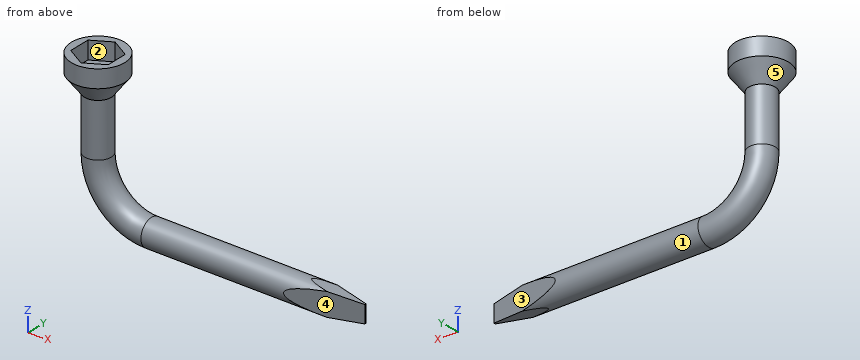
Autodesk Inventor part; units mm, degrees
ref_plane "YZ Plane" through (0, 0, 0) normal (1, 0, 0) x (0, 1, 0)
ref_plane "XZ Plane" through (0, 0, 0) normal (0, 1, 0) x (-1, 0, 0)
ref_plane "XY Plane" through (0, 0, 0) normal (0, 0, 1) x (1, 0, 0)
sketch "Эскиз1" plane through (0, 0, 0) normal (0, 1, 0) x (-1, 0, 0)
  line L0 (0, 0) -> (0, -30)
  line L1 (-30, -60) -> (-150, -60)
  arc A0 (-30, -60) -> (0, -30) centre (-30, -30) ccw
  point P0 (0, -60)
  dimension "d0" = 60
  dimension "d1" = 150
  dimension "d2" = 30
sketch "Эскиз2" plane through (0, 0, 0) normal (0, 0, 1) x (1, 0, 0)
  circle A0 centre (0, 0) radius 7.5
  dimension "d3" = 15
sweep "Сдвиг1" add profiles "Эскиз2" path "Эскиз1"
sketch "Эскиз3" plane through (0, 0, 0) normal (0, 1, 0) x (-1, 0, 0)
  line L0 (-120, -52.5) -> (-150, -55.1247)
  line L1 (-120, -67.5) -> (-150, -64.8753)
  line L2 (-150, -64.8753) -> (-150, -55.1247)
  line L3 (-150, -52.5) -> (-150, -67.5)
  line L4 (-120, -52.5) -> (-150.8821, -45.0422)
  line L5 (-150.8821, -45.0422) -> (-158.2895, -61.433)
  line L6 (-158.2895, -61.433) -> (-150, -78.5011)
  line L7 (-150, -78.5011) -> (-120, -67.5)
  point P0 (0, 0)
extrude "Выдавливание1" cut sketch "Эскиз3" against normal mid plane 40
sketch "Эскиз4" plane through (0, 0, 0) normal (0, 0, 1) x (1, 0, 0)
  line L0 (30, 7.5) -> (150, 7.5)
  line L1 (110, 7.5) -> (150.3931, 7.5) construction
  line L2 (30, -7.5) -> (150, -7.5)
  line L3 (110, 7.5) -> (159.1062, 20.8998)
  line L4 (159.1062, 20.8998) -> (172.0854, -18.5057)
  line L5 (172.0854, -18.5057) -> (124.0272, -32.5373)
  line L6 (124.0272, -32.5373) -> (110, -7.5)
  line L7 (110, 7.5) -> (150, 0.4469)
  line L8 (150, -5.6992) -> (150, 5.6992)
  line L9 (110, 7.5) -> (150.6171, 7.5) construction
  line L10 (110, -7.5) -> (150, -0.4469)
  line L11 (150, 0.4469) -> (150, -0.4469)
  point P0 (0, 0)
  dimension "d13" = 10
extrude "Выдавливание2" cut sketch "Эскиз4" against normal blind 120
sketch "Эскиз5" plane through (0, 0, 0) normal (0, 1, 0) x (-1, 0, 0)
  line L0 (0, 0) -> (0, 20)
  line L1 (0, 20) -> (15, 20)
  line L2 (15, 20) -> (15, 10)
  line L3 (7.5, 0) -> (-7.5, 0)
  line L4 (7.5, 0) -> (15, 10)
  dimension "d14" = 20
  dimension "d15" = 15
  dimension "d16" = 10
revolve "Вращение1" add sketch "Эскиз5" angle 360 about axis through (0, 0, 0) along (0, 0, 1)
sketch "Эскиз10" plane through (0, 0, 20) normal (0, 0, 1) x (1, 0, 0)
  line L0 (0, 12.1042) -> (10.4826, 6.0521)
  line L1 (10.4826, 6.0521) -> (10.4826, -6.0521)
  line L2 (10.4826, -6.0521) -> (0, -12.1042)
  line L3 (0, -12.1042) -> (-10.4826, -6.0521)
  line L4 (-10.4826, -6.0521) -> (-10.4826, 6.0521)
  line L5 (-10.4826, 6.0521) -> (0, 12.1042)
  point P0 (0, 0)
  point P1 (0, 0)
extrude "Выдавливание3" cut sketch "Эскиз10" against normal blind 10
properties part number "ключ" material "Сталь, гальванизированная"
Verification items for the finished model (mm, model axes). Face numbers are marked on the shaded views. A direction names the side the tool comes from. Round coordinates to 2 decimals unless told otherwise and drop trailing zeros. Order: outer loops, then holes, each group sorted by start corner. A loop starts at its lowest first (then second) coordinate and runs counter-clockwise, first axis right, second up.
1) Depth check by flat-ended pin: pin 1 (8 mm diameter, centred on y = -5, z = 0, fed in from +X); pin 2 (12 mm diameter, centred on x = 117, z = -58.5, fed in from -Y); pin 3 (5 mm diameter, centred on y = 3, z = 13, fed in from +X); pin 4 (11 mm diameter, centred on y = 0.5, z = 17, fed in from -X). Enter the tip coordinate at first touch or a pass-through.
Geometry says:
pin 1: stops at x = 9.67
pin 2: stops at y = -7.32
pin 3: stops at x = 14.99
pin 4: stops at x = -15
2) Cross-section at A-A, the plane z = 6. Record the cut outline in (x, y), plus the area to 3 significant figures.
Geometry says:
outline: circle Ø24 at (0, 0)
area: 452 mm2
3) Cross-section at B-B, the plane x = 32. Record the cut outline in (y, z).
Geometry says:
outline: circle Ø15 at (0, -60)
4) Material ranges on line 1 (Y direction, x = 33.5, z = -60.5); line 2 (Z direction, x = 37, y = -3.75); line 3 (X direction, y = 3, z = 13), recorded low to high.
Geometry says:
line 1: y = -7.48 to 7.48
line 2: z = -66.5 to -53.5
line 3: x = -14.7 to -10.48, 10.48 to 14.7
5) Draft check along X on the marked faces 1, 2 and 3. Enter one of: +X half, -X half, draft (parallel to the pull), parting line (faces both ways), or undercut.
Geometry says:
face 1: draft
face 2: undercut
face 3: +X half
6) Tool access check on the marked faces 4 and 5. Record the directions out of +Z, -Z, +X, -X, +Y, -Y that give a thin tool (end or side, any length) a straight path to the whole face; none if there is none.
Geometry says:
face 4: +Z, -Z, +X, -Y
face 5: none
